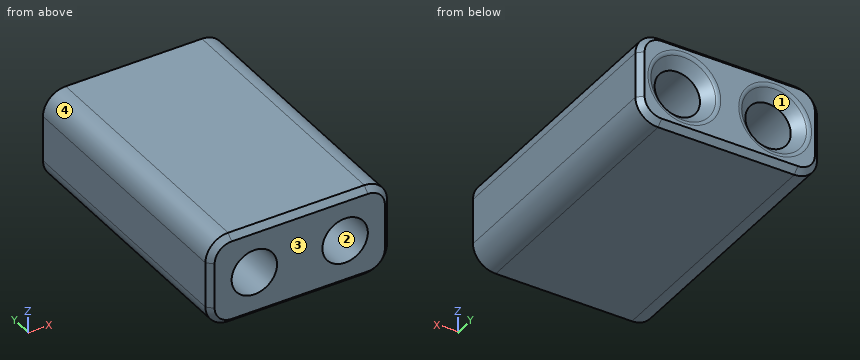
```python
from build123d import *

# Parameters (mm, degrees)
F0_W     = 16
F0_H     = 24
F1_DEPTH = 8
F2_R     = 2
F3_DEPTH = 50
F5_R     = 2
F6_SIZE  = 0.5
F7_SIZE  = 1
F8_R     = 0.5


with BuildPart() as f1:
    # F0 (on Top) → F1 (new body)
    with BuildSketch(Plane.XY):
        Rectangle(F0_W, F0_H)
    extrude(amount=F1_DEPTH)

    # F2 (on face) → F3 (cut)
    with BuildSketch(Plane.XZ.offset(12)):
        with Locations((-4, 4)):
            Circle(F2_R)
    extrude(amount=-F3_DEPTH, mode=Mode.SUBTRACT)

    # F4: F1 across plane


with BuildPart() as f1_1:
    add(f1.part)
    add(f1.part.mirror(Plane.YZ), mode=Mode.INTERSECT)

    # F5
    f5_edges = [f1_1.edges().sort_by_distance(p)[0] for p in [
        (-8, 0, 8),
        (8, 0, 8),
        (8, 0, 0),
        (-8, 0, 0),
    ]]
    fillet(f5_edges, radius=F5_R)

    # F6
    f6_edges = [f1_1.edges().sort_by_distance(p)[0] for p in [
        (0, -12, 8),
        (0, 12, 8),
        (8, 12, 4),
        (7.414214, 12, 0.585786),
        (7.414214, 12, 7.414214),
        (0, 12, 0),
        (-7.414214, 12, 0.585786),
        (-7.414214, 12, 7.414214),
        (-8, 12, 4),
        (8, -12, 4),
        (7.414214, -12, 0.585786),
        (7.414214, -12, 7.414214),
        (0, -12, 0),
        (-7.414214, -12, 0.585786),
        (-7.414214, -12, 7.414214),
        (-8, -12, 4),
    ]]
    chamfer(f6_edges, length=F6_SIZE)

    # F7
    f7_edges = [f1_1.edges().sort_by_distance(p)[0] for p in [
        (6, 12, 4),
        (-6, 12, 4),
    ]]
    chamfer(f7_edges, length=F7_SIZE)

    # F8
    f8_edges = [f1_1.edges().sort_by_distance(p)[0] for p in [
        (-7, 12, 4),
        (7, 12, 4),
    ]]
    fillet(f8_edges, radius=F8_R)


solid = f1_1.part
```
Check sheet for the modelled part. Datum: model origin and axes. Units: mm. Face numbers are marked on the shaded views. Coordinates: 2 decimals unless noted, no trailing zeros. Order: outer loops, then holes, each group sorted by start corner. A loop starts at its lowest first (then second) coordinate and runs counter-clockwise, first axis right, second up. Notation, with made-up numbers: M -9.75,71.25 L 12.25,71.25 A8 cw 12.25,83.25 Z; hole C 8.25,63 d5. An arc over 180 degrees is marked long. One line per question, with ' | ' between items. Start each with the question number.
Item 1: Sectioned sample at C-C on z = 5.75. Count the separate pieces of the cut face and the enclosed holes in it, and give its area (3 significant figures).
Item 2: Gauge pin test, flat end, axial feed: P1, Ø3, axis at x = -4, z = 4, coming from the +Y side. Record the tip position at first contact, or that the pin passes through.
Item 3: Mould release check, pull along Z, two halves, no side actions. Record for the marked faces 1, 2, 3 and 4: pulls with the +Z half, pulls with the -Z half, needs draft (parallel to the pull), parting line crosses it, or undercut.
Item 4: Sectioned sample at B-B on y = -7. Record the cut outline in (x, z).
Item 5: Material ranges on line 1 (X direction, y = 9.25, z = 3); line 2 (X direction, y = -9.25, z = 3.5); line 3 (Z direction, x = -5.5, y = 0.25), recorded low to high.
Item 6: Sectioned sample at A-A on x = -4. Record the cut outline in (y, z), and give its area (3 significant figures).
Answer below:
1) separate pieces: 3 | enclosed holes: 0 | area: 287 mm^2
2) P1: passes through
3) face 1: undercut | face 2: undercut | face 3: needs draft | face 4: pulls with the +Z half
4) outline: M -8,2 A2 ccw -6,0 L 6,0 A2 ccw 8,2 L 8,6 A2 ccw 6,8 L -6,8 A2 ccw -8,6 Z; hole C -4,4 d4; hole C 4,4 d4
5) line 1: x = -8 to -5.73, -2.27 to 2.27, 5.73 to 8 | line 2: x = -8 to -5.94, -2.06 to 2.06, 5.94 to 8 | line 3: z = 0 to 2.68, 5.32 to 8
6) outline: M -12,0.5 L -11.5,0 L 11.5,0 L 12,0.5 L 12,0.79 A0.5 ccw 11.85,1.15 L 11,2 L -12,2 Z; M -12,6 L 11,6 L 11.85,6.85 A0.5 ccw 12,7.21 L 12,7.5 L 11.5,8 L -11.5,8 L -12,7.5 Z | area: 94.5 mm^2
